from build123d import *

# Parameters (mm, degrees)
SKETCH1_R           = 1
BOSS_EXTRUDE1_DEPTH = 53.2


with BuildPart() as part:
    # Sketch1 → Boss-Extrude1 (new body)
    with BuildSketch(Plane.XY):
        with BuildLine():
            Line((-23.7, 19.2), (-25.185156579, 19.199963279))
            ThreePointArc((-25.185156579, 19.199963279), (-27.316065894, 18.32656181), (-28.2, 16.2))
            Line((-28.2, 16.2), (-28.2, -16.2))
            ThreePointArc((-28.2, -16.2), (-27.316065894, -18.32656181), (-25.185156579, -19.199963279))
            Line((-25.185156579, -19.199963279), (-23.7, -19.2))
            ThreePointArc((-23.7, -19.2), (-20.518019485, -20.518019485), (-19.2, -23.7))
            Line((-19.2, -23.7), (-19.2, -25.2))
            ThreePointArc((-19.2, -25.2), (-18.321320344, -27.321320344), (-16.2, -28.2))
            Line((-16.2, -28.2), (16.2, -28.2))
            ThreePointArc((16.2, -28.2), (18.321320344, -27.321320344), (19.2, -25.2))
            Line((19.2, -25.2), (19.2, -23.7))
            ThreePointArc((19.2, -23.7), (20.518019485, -20.518019485), (23.7, -19.2))
            Line((23.7, -19.2), (25.185156579, -19.199963279))
            ThreePointArc((25.185156579, -19.199963279), (27.316065894, -18.32656181), (28.2, -16.2))
            Line((28.2, -16.2), (28.2, 16.2))
            ThreePointArc((28.2, 16.2), (27.316065894, 18.32656181), (25.185156579, 19.199963279))
            Line((25.185156579, 19.199963279), (23.7, 19.2))
            ThreePointArc((23.7, 19.2), (20.518019485, 20.518019485), (19.2, 23.7))
            Line((19.2, 23.7), (19.2, 25.2))
            ThreePointArc((19.2, 25.2), (18.321320344, 27.321320344), (16.2, 28.2))
            Line((16.2, 28.2), (-16.2, 28.2))
            ThreePointArc((-16.2, 28.2), (-18.321320344, 27.321320344), (-19.2, 25.2))
            Line((-19.2, 25.2), (-19.2, 23.7))
            ThreePointArc((-19.2, 23.7), (-20.518019485, 20.518019485), (-23.7, 19.2))
        make_face()
        with Locations((-25.2, 16.2)):
            Circle(SKETCH1_R, mode=Mode.SUBTRACT)
        with Locations((16.2, 25.2)):
            Circle(SKETCH1_R, mode=Mode.SUBTRACT)
        with Locations((25.2, -16.2)):
            Circle(SKETCH1_R, mode=Mode.SUBTRACT)
        with Locations((-16.2, -25.2)):
            Circle(SKETCH1_R, mode=Mode.SUBTRACT)
        Polygon((10.810973978, -26.1), (26.1, -10.810973978), (26.1, 10.810973978), (10.810973978, 26.1), (-10.810973978, 26.1), (-26.1, 10.810973978), (-26.1, -10.810973978), (-10.810973978, -26.1), align=None, mode=Mode.SUBTRACT)
    extrude(amount=BOSS_EXTRUDE1_DEPTH)


solid = part.part
Here's how the part is built. I have some questions about the finished solid (model axes, mm). A direction names the side the tool comes from. Coordinates: 2 decimals unless noted, no trailing zeros. Loops run counter-clockwise (first coordinate to the right, second up) from the corner with the lowest first, then second, coordinate; pieces in that order, holes last.
1. For faces 1 (the flat face through (19.2, 24, 26)), 2 (the cylindrical face through (18.3, -27.34, 26.23)), 3 (the flat face through (0, 26.1, 26)), which set-ups out of +Z, -Z, +X, -X, +Y, -Y let a thin tool reach every point of the face, with its end or its side?
2. Imagine slicing it at A-A, the plane y = 0.5. Please give me the cut outline in (x, z), and give its area (3 significant figures).
3. If we mould it in two halves opening along X, with no side actions, what happens to faces 4 (the flat face through (19.2, -24, 26)), 5 (the cylindrical face through (-18.34, -27.3, 26.23)), 6 (the flat face through (18.56, 18.35, 26.23))? For each: pulls with the +X half, pulls with the -X half, needs draft (parallel to the pull), parting line crosses it, or undercut.
4. I need wall thicknesses on L1, parallel to X at y = 16, z = 22; L2, parallel to Y at x = 8, z = 4. Which ranges of each line are inside material? Lowest first, please.
5. For P1, Ø0.8, axis at y = 25, z = 32.5, coming from the -X side; P2, Ø1.2, axis at y = 24, z = 13.5, coming from the +X side; P3, Ø0.7, axis at x = 24.5, z = 19.5, coming from the -Y side; P4, Ø1.6, axis at x = -25.2, y = 16.2, coming from the -Z side, each with a flat end and sliding along its axis, tell me the tip position at first contact or that it passes through.
6. Imagine slicing it at B-B, the plane z = 4.5. Count the separate pieces of the cut face and the enclosed holes in it, and give its area (3 significant figures).
Taken from the geometry:
1. face 1: +Z, -Z, +X, +Y
1. face 2: +Z, -Z, +X, -Y
1. face 3: +Z, -Z
2. outline: (-28.2, 0) - (-26.1, 0) - (-26.1, 53.2) - (-28.2, 53.2) - close; (26.1, 0) - (28.2, 0) - (28.2, 53.2) - (26.1, 53.2) - close
2. area: 223 mm2
3. face 4: pulls with the +X half
3. face 5: pulls with the -X half
3. face 6: undercut
4. L1: x = -28.2 to -26.18, -24.22 to -20.91, 20.91 to 28.2
4. L2: y = -28.2 to -26.1, 26.1 to 28.2
5. P1: stops at x = -19.2
5. P2: stops at x = 19.21
5. P3: stops at y = -19.2
5. P4: passes through
6. separate pieces: 1
6. enclosed holes: 5
6. area: 589 mm2
